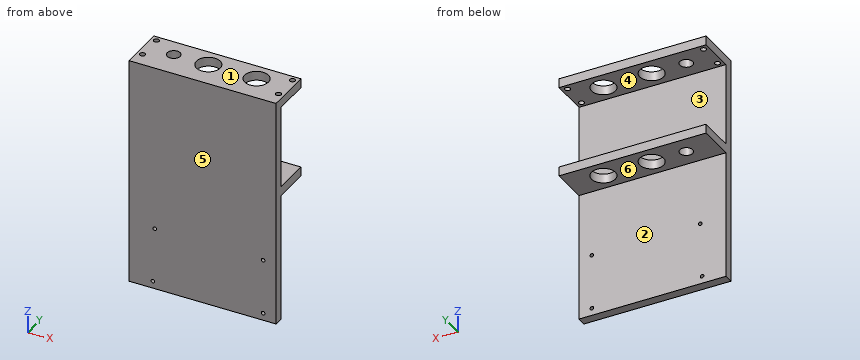
```python
from build123d import *

# Parameters (mm, degrees)
SKETCH_1_W               = 80
SKETCH_1_H               = 25
EXTRUDE_1_DEPTH          = 5
SKETCH_2_W               = 80
SKETCH_2_H               = 5
EXTRUDE_2_DEPTH          = 120
SKETCH_3_W               = 80
SKETCH_3_H               = 5
EXTRUDE_3_DEPTH          = 20
SKETCH_4_R               = 1.5
CUT_EXTRUDE_1_DEPTH      = 20
SKETCH_5_R               = 6.5
CUT_EXTRUDE_2_DEPTH      = 121
CUT_EXTRUDE_2_DEPTH_BACK = 6
SKETCH_6_R               = 3.5
CUT_EXTRUDE_3_DEPTH      = 121
CUT_EXTRUDE_3_DEPTH_BACK = 6
SKETCH_7_R               = 1
CUT_EXTRUDE_4_DEPTH      = 20


with BuildPart() as part:
    # 스케치1 → 보스-돌출1 (new body)
    with BuildSketch(Plane.XY):
        with Locations((40, 12.5)):
            Rectangle(SKETCH_1_W, SKETCH_1_H)
    extrude(amount=EXTRUDE_1_DEPTH)

    # 스케치2 → 보스-돌출2 (add)
    with BuildSketch(Plane(origin=(0, 0, 0), x_dir=(-1, 0, 0), z_dir=(0, 0, -1))):
        with Locations((-40, 2.5)):
            Rectangle(SKETCH_2_W, SKETCH_2_H)
    extrude(amount=EXTRUDE_2_DEPTH)

    # 스케치3 → 보스-돌출3 (add)
    with BuildSketch(Plane(origin=(0, 5, 0), x_dir=(1, 0, 0), z_dir=(0, 1, 0))):
        with Locations((40, 47.5)):
            Rectangle(SKETCH_3_W, SKETCH_3_H)
    extrude(amount=EXTRUDE_3_DEPTH)

    # 스케치4 → 컷-돌출1 (cut)
    with BuildSketch(Plane(origin=(0, 0, 0), x_dir=(-1, 0, 0), z_dir=(0, 0, -1))):
        with Locations((-77, 22)):
            Circle(SKETCH_4_R)
        with Locations((-77, 8)):
            Circle(SKETCH_4_R)
        with Locations((-3, 22)):
            Circle(SKETCH_4_R)
        with Locations((-3, 8)):
            Circle(SKETCH_4_R)
    extrude(amount=-CUT_EXTRUDE_1_DEPTH, mode=Mode.SUBTRACT)

    # 스케치5 → 컷-돌출2 (cut, two sides)
    with BuildSketch(Plane(origin=(0, 0, 0), x_dir=(-1, 0, 0), z_dir=(0, 0, -1))) as cut_extrude_2_sk:
        with Locations((-61.258324532, 15)):
            Circle(SKETCH_5_R)
        with Locations((-35.004725497, 15)):
            Circle(SKETCH_5_R)
    extrude(amount=CUT_EXTRUDE_2_DEPTH, mode=Mode.SUBTRACT)
    extrude(cut_extrude_2_sk.sketch, amount=-CUT_EXTRUDE_2_DEPTH_BACK, mode=Mode.SUBTRACT)

    # 스케치6 → 컷-돌출3 (cut, two sides)
    with BuildSketch(Plane(origin=(0, 0, 0), x_dir=(-1, 0, 0), z_dir=(0, 0, -1))) as cut_extrude_3_sk:
        with Locations((-16.191806112, 15)):
            Circle(SKETCH_6_R)
    extrude(amount=CUT_EXTRUDE_3_DEPTH, mode=Mode.SUBTRACT)
    extrude(cut_extrude_3_sk.sketch, amount=-CUT_EXTRUDE_3_DEPTH_BACK, mode=Mode.SUBTRACT)

    # 스케치7 → 컷-돌출4 (cut)
    with BuildSketch(Plane(origin=(0, 5, 0), x_dir=(1, 0, 0), z_dir=(0, 1, 0))):
        with Locations((73, 116)):
            Circle(SKETCH_7_R)
        with Locations((73, 86)):
            Circle(SKETCH_7_R)
        with Locations((13, 116)):
            Circle(SKETCH_7_R)
        with Locations((14, 86)):
            Circle(SKETCH_7_R)
    extrude(amount=-CUT_EXTRUDE_4_DEPTH, mode=Mode.SUBTRACT)


solid = part.part
```
Input: part model. Units: mm. Frame: model coordinates. Face numbers are marked on the shaded views. A direction names the side the tool comes from. Give positions to 0.01 mm unless a question says otherwise; leave off trailing zeros. Order: outer loops, then holes, each group sorted by start corner. A loop starts at its lowest first (then second) coordinate and runs counter-clockwise, first axis right, second up.
1. Pin query (flat end, axial travel): pin 1 (10 mm diameter, centred on x = 65.5, z = -98.5, fed in from -Y); pin 2 (5.5 mm diameter, centred on x = 16.19, y = 15, fed in from -Z); pin 3 (2 mm diameter, centred on x = 24.5, z = -71, fed in from +Y); pin 4 (8 mm diameter, centred on x = 67.5, y = 11, fed in from -Z). Return the tip coordinate at first contact, or that it passes through.
Derived:
pin 1: stops at y = 0
pin 2: passes through
pin 3: stops at y = 5
pin 4: stops at z = -50
2. Material intervals for L1, parallel to X at y = 1.7, z = -86; L2, parallel to Y at x = 3, z = 3.2; L3, parallel to X at y = 2.4, z = -116, sorted ascending.
Derived:
L1: x = 0 to 13, 15 to 72, 74 to 80
L2: y = 0 to 6.5, 9.5 to 20.5, 23.5 to 25
L3: x = 0 to 12, 14 to 72, 74 to 80
3. Section C-C on z = -105. Return the cut outline in (x, y).
Derived:
outline: (0, 0) - (80, 0) - (80, 5) - (0, 5) - close
4. Mould query, pull axis Z, two halves, no side actions, for the marked faces 1, 2 and 3. Classes: released by +Z, released by -Z, zero draft, split by the parting line, or undercut.
Derived:
face 1: released by +Z
face 2: zero draft
face 3: undercut
5. Section B-B on x = 50.5. Return the cut outline in (y, z), and give its area (3 significant figures).
Derived:
outline: (0, -120) - (5, -120) - (5, -50) - (25, -50) - (25, -45) - (5, -45) - (5, 0) - (25, 0) - (25, 5) - (0, 5) - close
area: 825 mm2
6. Section A-A on y = 15. Give the number of separate pieces and of enclosed holes in the cut face, and give its area (3 significant figures).
Derived:
separate pieces: 8
enclosed holes: 0
area: 470 mm2
7. Reachability of the marked faces 4, 5 and 6 from +Z, -Z, +X, -X, +Y, -Y: full face, straight path, thin tool, end or side. Return the list, or none.
Derived:
face 4: +X, -X, +Y
face 5: +Z, -Z, +X, -X, -Y
face 6: -Z, +X, -X, +Y
